Can you work these out from the model? Positions are in its coordinate system, mm. Face numbers are marked on the shaded views. A direction names the side the tool comes from. Give positions to 0.01 mm unless a question says otherwise; leave off trailing zeros. Loops run counter-clockwise (first coordinate to the right, second up) from the corner with the lowest first, then second, coordinate; pieces in that order, holes last. Notation, with made-up numbers: (9, -33) -> (54, -33) arc R25 ccw to (54, -5) -> close; hole circle Ø10 at (86.25, 27.5). An arc over 180 degrees is marked (long way). Return JSON: item names as keys, results as strings. Group by question number.
Q1. Which directions (+Z, -Z, +X, -X, +Y, -Y) give clear straight access to the entire face, cutting with the end or side of a thin tool? Please do the marked faces 1, 2, 3 and 4.
Q2. Suppose I cut it at D-D, the plane x = 19. Please give me the cut outline in (y, z).
Q3. Suppose I cut it at A-A, the plane x = 23. Please give me the cut outline in (y, z).
Q4. Thinking about a two-plate mould opening in Y: for the marked faces 5, 6 and 7, which applies, pulls with the +Y half, pulls with the -Y half, needs draft (parallel to the pull), parting line crosses it, or undercut?
Q5. Suppose I cut it at C-C, the plane z = 20.5. Please give me the cut outline in (x, y), and give its area (3 significant figures).
Q6. I need wall thicknesses on line 1 along Z through (x, y) = (9.75, 13); line 2 along X through (y, z) = (7, 17); line 3 along Z through (x, y) = (16.75, 6). Which ranges of each line are inside material? Lowest first, please. Write a range as [from, to].
Q7. Suppose I cut it at B-B, the plane z = -17.5. Please give me the cut outline in (x, y).
Q8. Will these pins go through, and if not, where does the flat tip stop? pin 1 (5 mm diameter, centred on x = 15.65, z = 17.5, fed in from +Y); pin 2 (5 mm diameter, centred on x = 23, z = -17.5, fed in from -Y); pin 3 (3 mm diameter, centred on x = 7.5, z = 5.5, fed in from +Y); pin 4 (12 mm diameter, centred on x = 3, z = 11, fed in from +Y).
```python
from build123d import *

# Parameters (mm, degrees)
BOSS_EXTRUDE1_DEPTH          = 22.5
CUT_EXTRUDE1_START           = -28
SKETCH12_W                   = 25
SKETCH12_H                   = 9
CUT_EXTRUDE1_DEPTH           = 16
CUT_EXTRUDE2_START           = -28
SKETCH13_R                   = 1.75
CUT_EXTRUDE2_DEPTH           = 10
CUT_EXTRUDE2_DRAFT           = 6
CUT_EXTRUDE2_PROFILE_2_DEPTH = 10
CUT_EXTRUDE2_PROFILE_2_DRAFT = 6
FILLET1_R                    = 7
FILLET2_R                    = 1
SKETCH17_R                   = 1.6
CUT_EXTRUDE5_DEPTH           = 46.543934832


# Read off the part's stored shape, not the designer's step: Cut-Extrude3
with BuildPart() as part:
    # Sketch1 → Boss-Extrude1 (new, symmetric)
    with BuildSketch(Plane.XY):
        Polygon((10, 16), (28, 16), (28, 0), (10, 0), (10, -12), (0, -12), (0, 0), (0, 21), align=None)
    extrude(amount=BOSS_EXTRUDE1_DEPTH, both=True)

    # Sketch12 → Cut-Extrude1 (cut)
    with BuildSketch(Plane(origin=(28, 0, 0), x_dir=(0, 0, -1), z_dir=(1, 0, 0)).offset(CUT_EXTRUDE1_START)):
        with Locations((0, 4.5)):
            Rectangle(SKETCH12_W, SKETCH12_H)
    extrude(amount=CUT_EXTRUDE1_DEPTH, mode=Mode.SUBTRACT)


with BuildPart() as cut_extrude2_tool:
    # Sketch13 → Cut-Extrude2 (with draft: the straight prism first)
    with BuildSketch(Plane(origin=(28, 0, 0), x_dir=(0, 0, -1), z_dir=(1, 0, 0)).offset(CUT_EXTRUDE2_START)):
        with Locations((11.7, 12.996154984)):
            Circle(SKETCH13_R)
    extrude(amount=CUT_EXTRUDE2_DEPTH)
    # Cut-Extrude2: the draft: its side faces are tilted about the plane it starts from
    cut_extrude2_sides = [cut_extrude2_tool.faces().sort_by_distance(p)[0] for p in [
        (5, 12.996154984, -9.95),
    ]]
    draft(cut_extrude2_sides, Plane(origin=(28, 0, 0), x_dir=(0, 0, -1), z_dir=(1, 0, 0)).offset(CUT_EXTRUDE2_START), CUT_EXTRUDE2_DRAFT)


with BuildPart() as part_1:
    add(part.part)

    # Cut-Extrude2: cut by cut_extrude2_tool
    add(cut_extrude2_tool.part, mode=Mode.SUBTRACT)


with BuildPart() as cut_extrude2_profile_2_tool:
    # Sketch13 → Cut-Extrude2 profile 2 (with draft: the straight prism first)
    with BuildSketch(Plane(origin=(28, 0, 0), x_dir=(0, 0, -1), z_dir=(1, 0, 0)).offset(CUT_EXTRUDE2_START)):
        with Locations((-11.7, 12.996154984)):
            Circle(SKETCH13_R)
    extrude(amount=CUT_EXTRUDE2_PROFILE_2_DEPTH)
    # Cut-Extrude2 profile 2: the draft: its side faces are tilted about the plane it starts from
    cut_extrude2_profile_2_sides = [cut_extrude2_profile_2_tool.faces().sort_by_distance(p)[0] for p in [
        (5, 12.996154984, 13.45),
    ]]
    draft(cut_extrude2_profile_2_sides, Plane(origin=(28, 0, 0), x_dir=(0, 0, -1), z_dir=(1, 0, 0)).offset(CUT_EXTRUDE2_START), CUT_EXTRUDE2_PROFILE_2_DRAFT)


with BuildPart() as part_2:
    add(part_1.part)

    # Cut-Extrude2 profile 2: cut by cut_extrude2_profile_2_tool
    add(cut_extrude2_profile_2_tool.part, mode=Mode.SUBTRACT)

    # Cut-Extrude3 outline → Cut-Extrude3 (revolve, cut)
    with BuildSketch(Plane(origin=(0, -4.753845016, 11.7), x_dir=(0, 1, 0), z_dir=(0, 0, -1))):
        Polygon((0, 0), (1.75, 0), (0.522154391, 10), (0, 10), align=None)
    revolve(axis=Axis((0, -4.753845016, 11.7), (1, 0, 0)), mode=Mode.SUBTRACT)

    # Cut-Extrude3 2 outline → Cut-Extrude3 2 (revolve, cut)
    with BuildSketch(Plane(origin=(0, -4.753845016, -11.7), x_dir=(0, 1, 0), z_dir=(0, 0, -1))):
        Polygon((0, 0), (1.75, 0), (0.522154391, 10), (0, 10), align=None)
    revolve(axis=Axis((0, -4.753845016, -11.7), (1, 0, 0)), mode=Mode.SUBTRACT)

    # Fillet1
    fillet1_edges = [part_2.edges().sort_by_distance(p)[0] for p in [
        (10, 16, 0),
    ]]
    fillet(fillet1_edges, radius=FILLET1_R)

    # Fillet2
    fillet2_edges = [part_2.edges().sort_by_distance(p)[0] for p in [
        (5, -12, -22.5),
        (28, 16, 0),
        (0, -12, 0),
        (0, 21, 0),
        (5, -12, 22.5),
        (28, 8, 22.5),
        (19.826237921, 16, 22.5),
        (4.260990337, 18.869504832, -22.5),
        (4.260990337, 18.869504832, 22.5),
        (10.044205399, 16.187257074, -22.5),
        (10.044205399, 16.187257074, 22.5),
        (19.826237921, 16, -22.5),
        (28, 8, -22.5),
    ]]
    fillet(fillet2_edges, radius=FILLET2_R)

    # Sketch17 → Cut-Extrude5 (cut, through all)
    with BuildSketch(Plane(origin=(0, 16, 0), x_dir=(1, 0, 0), z_dir=(0, 1, 0))):
        with Locations(Location((23, 17.5, 0), (0, 0, 270))):
            Circle(SKETCH17_R)
        with Locations(Location((15.652475842, 17.5, 0), (0, 0, 180))):
            Circle(SKETCH17_R)
        with Locations(Location((15.652475842, -17.5, 0), (0, 0, 270))):
            Circle(SKETCH17_R)
        with Locations(Location((23, -17.5, 0), (0, 0, 180))):
            Circle(SKETCH17_R)
    extrude(amount=-CUT_EXTRUDE5_DEPTH, mode=Mode.SUBTRACT)


solid = part_2.part
```
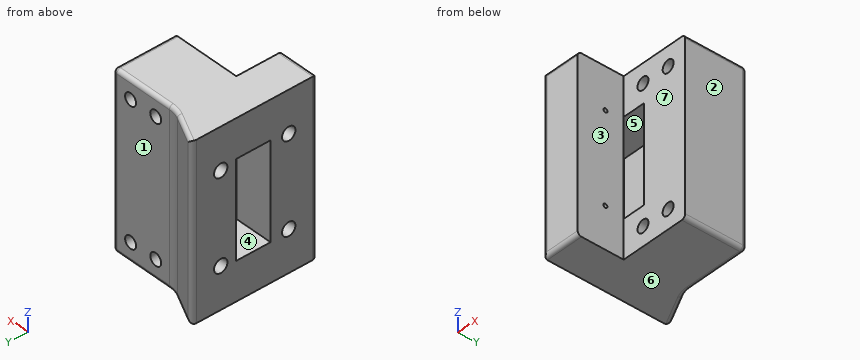
Ans:
{
 "1": {"face 1": "+Z, -Z, +X, +Y", "face 2": "+Z, -Z, +X, +Y, -Y", "face 3": "+Z, -Z, +X, -Y", "face 4": "-X"},
 "2": {"outline": "(0, -22.5) -> (15, -22.5) arc R1 ccw to (16, -21.5) -> (16, 21.5) arc R1 ccw to (15, 22.5) -> (0, 22.5) -> close"},
 "3": {"outline": "(0, -22.5) -> (15, -22.5) arc R1 ccw to (16, -21.5) -> (16, -19.1) -> (0, -19.1) -> close; (0, -15.9) -> (16, -15.9) -> (16, 15.9) -> (0, 15.9) -> close; (0, 19.1) -> (16, 19.1) -> (16, 21.5) arc R1 ccw to (15, 22.5) -> (0, 22.5) -> close"},
 "4": {"face 5": "undercut", "face 6": "needs draft", "face 7": "pulls with the -Y half"},
 "5": {"outline": "(0, -11) arc R1 ccw to (1, -12) -> (10, -12) -> (10, 0) -> (28, 0) -> (28, 15) arc R1 ccw to (27, 16) -> (11.65, 16) arc R7 cw to (8.52, 16.74) -> (1.45, 20.28) arc R1 ccw to (0, 19.38) -> close", "area": "592 mm^2"},
 "6": {"line 1": "z = [-22.5, -12.43], [-10.97, 10.97], [12.43, 22.5]", "line 2": "x = [0, 14.13], [17.17, 21.48], [24.52, 28]", "line 3": "z = [-22.5, -18.66], [-16.34, 16.34], [18.66, 22.5]"},
 "7": {"outline": "(0, -11) arc R1 ccw to (1, -12) -> (10, -12) -> (10, 0) -> (14.05, 0) -> (14.05, 16) -> (11.65, 16) arc R7 cw to (8.52, 16.74) -> (1.45, 20.28) arc R1 ccw to (0, 19.38) -> close; (17.25, 0) -> (21.4, 0) -> (21.4, 16) -> (17.25, 16) -> close; (24.6, 0) -> (28, 0) -> (28, 15) arc R1 ccw to (27, 16) -> (24.6, 16) -> close"},
 "8": {"pin 1": "stops at y = 16", "pin 2": "stops at y = 0", "pin 3": "stops at y = 18", "pin 4": "stops at y = 20.38"}
}
